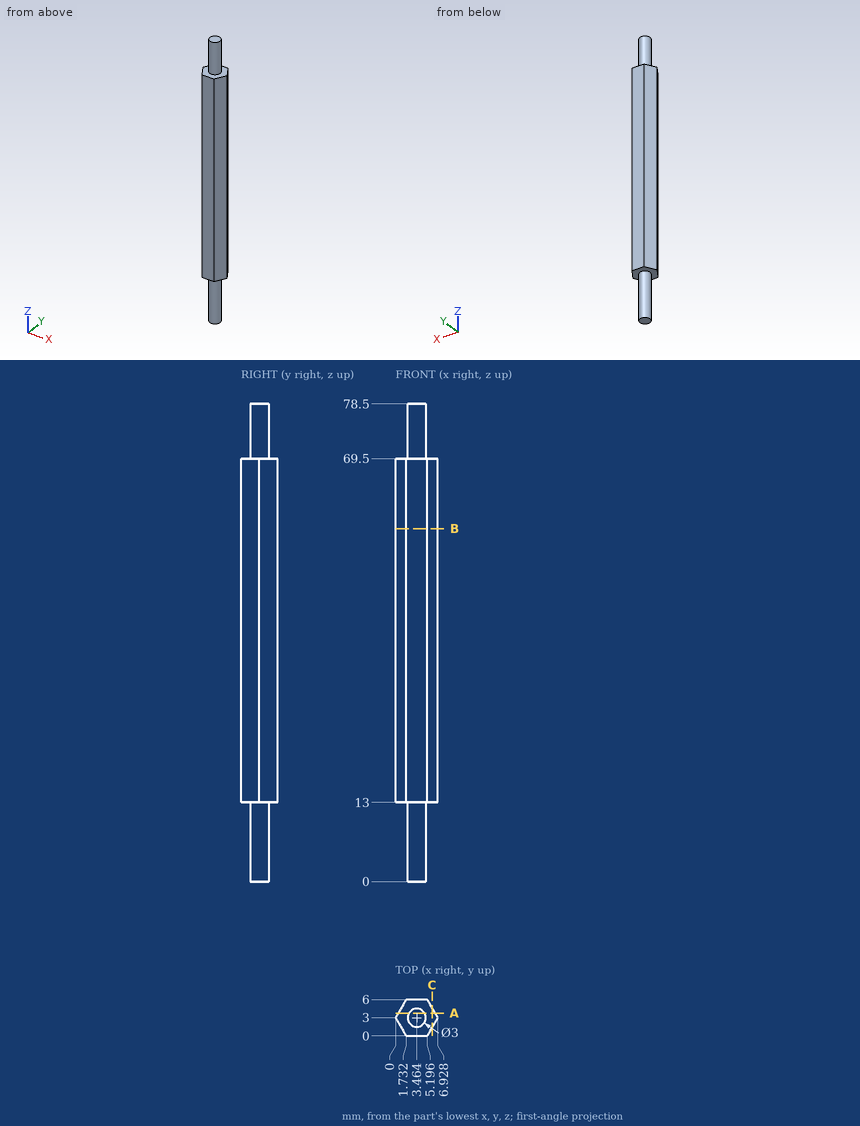
Job drawing, mm, ordinate dimensions from the low corner. One solid piece. Coordinates: 2 decimals unless noted, no trailing zeros. Loops run counter-clockwise (first coordinate to the right, second up) from the corner with the lowest first, then second, coordinate; pieces in that order, holes last. Notation, with made-up numbers: (37.5, 44) -> (52.5, 44) arc R23 cw to (52.5, 58) -> close; hole circle Ø4 at (-21.5, 27). An arc over 180 degrees is marked (long way). One line per item, written item: value.
1. Slice it at C-C on x = 6. Write the cut outline in (y, z), and give its area (3 significant figures).
Answers:
outline: (1.39, 13) -> (4.61, 13) -> (4.61, 69.5) -> (1.39, 69.5) -> close
area: 182 mm^2
2. Slice it at B-B on z = 58. Write the cut outline in (x, y).
Answers:
outline: (0, 3) -> (1.73, 0) -> (5.2, 0) -> (6.93, 3) -> (5.2, 6) -> (1.73, 6) -> close
3. Flat gauge pin, fed straight in: P1, Ø1.5, axis at y = 3.5, z = 8, coming from the -X side. Where does the tip first touch, or does it go through?
Answers:
P1: stops at x = 1.96
4. Drill centre lines: line 1 (Z direction, x = 4, y = 4.75); line 2 (X direction, y = 1.75, z = 46); line 3 (X direction, y = 5.5, z = 43) (1 decimal). Where is each one in solid material? Low to high. Write a range as [from, to].
Answers:
line 1: z = [13, 69.5]
line 2: x = [0.72, 6.21]
line 3: x = [1.4, 5.5]
5. Slice it at A-A on y = 3.75. Write the cut outline in (x, z) (1 decimal).
Answers:
outline: (0.4, 13) -> (2.2, 13) -> (2.2, 0) -> (4.8, 0) -> (4.8, 13) -> (6.5, 13) -> (6.5, 69.5) -> (4.8, 69.5) -> (4.8, 78.5) -> (2.2, 78.5) -> (2.2, 69.5) -> (0.4, 69.5) -> close
